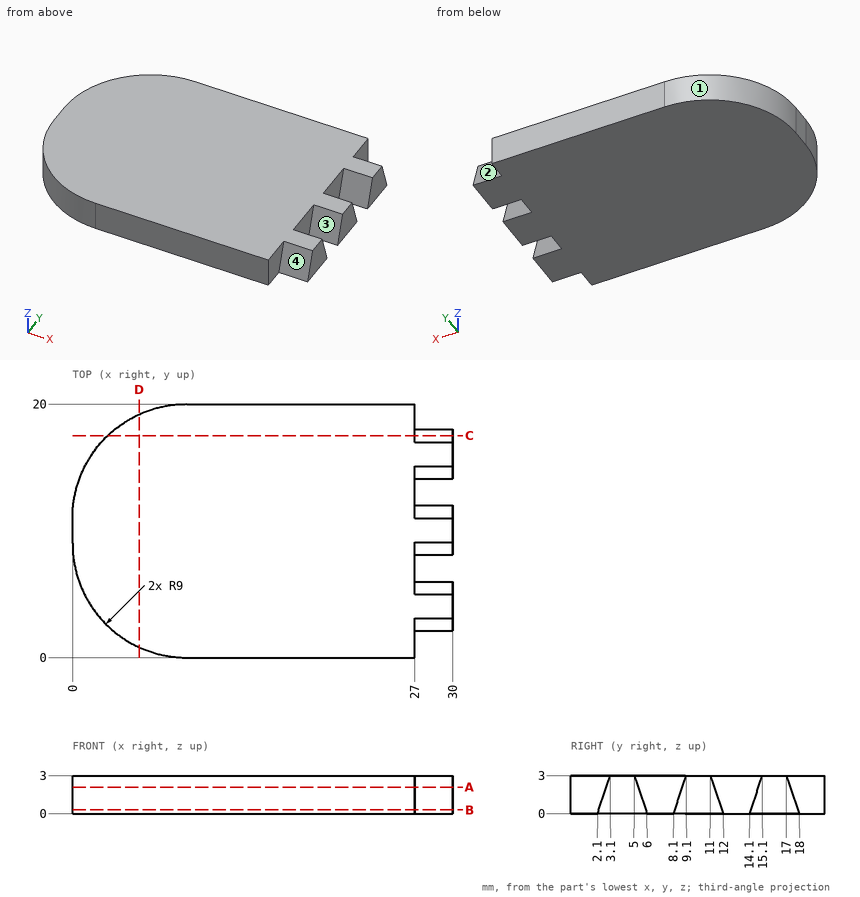
Study the drawing (mm; zero at the part's minimum x, y, z) and answer. A direction names the side the tool comes from. Coordinates: 2 decimals unless noted, no trailing zeros. Order: outer loops, then holes, each group sorted by start corner. A loop starts at its lowest first (then second) coordinate and runs counter-clockwise, first axis right, second up. Notation, with made-up numbers: (85, 24) -> (139, 24) arc R18 ccw to (139, 30) -> close; hole circle Ø10 at (-5, -10). An arc over 180 degrees is marked (long way). Answer in a Markdown table with one row per item. Add a question column.
Item 1: Which of the six approach directions +Z, -Z, +X, -X, +Y, -Y give full straight-line access (tool end or side, diameter ignored) to the marked faces 1, 2, 3 and 4?
Item 2: Find section C-C (y = 17.5). Write down the section's boundary in (x, z), then the cut area to 3 significant figures.
Item 3: Find section B-B (z = 0.3). Write down the section's boundary in (x, y).
Item 4: Find section A-A (z = 2.1). Write down the section's boundary in (x, y).
Item 5: Find the intervals of material crossed by L1, parallel to Y at x = 28.5, z = 0.4; L2, parallel to X at y = 4, z = 0.6; L3, parallel to X at y = 4.5, z = 1.35, in increasing order. Write a range as from..to.
Item 6: This flat-tipped pin is pushed along its axis until it touches: P1, Ø1.5, axis at y = 13.5, z = 2, coming from the +X side. Where does it stop, or does it pass through?
Item 7: Find section D-D (x = 5.25). Write down the section's boundary in (y, z).
Result set:
| question | item | result |
|---|---|---|
| 1 | face 1 | +Z, -Z, -X, +Y |
| 1 | face 2 | +Z, +X, +Y |
| 1 | face 3 | +Z, +X |
| 1 | face 4 | +Z, +X, -Y |
| 2 | outline | (2.78, 0) -> (30, 0) -> (30, 1.5) -> (27, 1.5) -> (27, 3) -> (2.78, 3) -> close |
| 2 | area | 77.2 mm² |
| 3 | outline | (0, 9) arc R9 ccw to (9, 0) -> (27, 0) -> (27, 2.2) -> (30, 2.2) -> (30, 5.9) -> (27, 5.9) -> (27, 8.2) -> (30, 8.2) -> (30, 11.9) -> (27, 11.9) -> (27, 14.2) -> (30, 14.2) -> (30, 17.9) -> (27, 17.9) -> (27, 20) -> (9, 20) arc R9 ccw to (0, 11) -> close |
| 4 | outline | (0, 9) arc R9 ccw to (9, 0) -> (27, 0) -> (27, 2.8) -> (30, 2.8) -> (30, 5.3) -> (27, 5.3) -> (27, 8.8) -> (30, 8.8) -> (30, 11.3) -> (27, 11.3) -> (27, 14.8) -> (30, 14.8) -> (30, 17.3) -> (27, 17.3) -> (27, 20) -> (9, 20) arc R9 ccw to (0, 11) -> close |
| 5 | L1 | y = 2.23..5.87, 8.23..11.87, 14.23..17.87 |
| 5 | L2 | x = 1.52..30 |
| 5 | L3 | x = 1.21..30 |
| 6 | P1 | stops at x = 27 |
| 7 | outline | (0.82, 0) -> (19.18, 0) -> (19.18, 3) -> (0.82, 3) -> close |
